Verification items for the finished model (mm, model axes). A direction names the side the tool comes from. Round coordinates to 2 decimals unless told otherwise and drop trailing zeros. Order: outer loops, then holes, each group sorted by start corner. A loop starts at its lowest first (then second) coordinate and runs counter-clockwise, first axis right, second up. Notation, with made-up numbers: M 70,63.5 L 92,63.5 A6 cw 92,74.5 Z; hole C -26,48 d4. An arc over 180 degrees is marked long. Return JSON: item names as keys, results as strings. Group by question number.
from build123d import *

# Parameters (mm, degrees)
BOSS_EXTRU_1_DEPTH      = 530
ESQUISSE2_R             = 2.5
ENL_V_MAT_EXTRU_1_DEPTH = 9


with BuildPart() as part:
    # Esquisse1 → Boss.-Extru.1 (new body)
    with BuildSketch(Plane.XY):
        Polygon((0, 0), (90, 0), (90, 7), (49.5, 7), (49.5, 60), (40.5, 60), (40.5, 7), (0, 7), align=None)
    extrude(amount=BOSS_EXTRU_1_DEPTH)

    # Esquisse2 → Enlèv. mat.-Extru.1 (cut)
    with BuildSketch(Plane.ZY.offset(-40.5)):
        with Locations(Location((80, 50, 0), (0, 0, 270))):
            Circle(ESQUISSE2_R)
        with Locations(Location((80, 26, 0), (0, 0, 90))):
            Circle(ESQUISSE2_R)
        with Locations(Location((180, 50, 0), (0, 0, 270))):
            Circle(ESQUISSE2_R)
        with Locations(Location((180, 26, 0), (0, 0, 90))):
            Circle(ESQUISSE2_R)
        with Locations(Location((280, 50, 0), (0, 0, 270))):
            Circle(ESQUISSE2_R)
        with Locations(Location((280, 26, 0), (0, 0, 90))):
            Circle(ESQUISSE2_R)
        with Locations(Location((380, 50, 0), (0, 0, 270))):
            Circle(ESQUISSE2_R)
        with Locations(Location((380, 26, 0), (0, 0, 90))):
            Circle(ESQUISSE2_R)
        with Locations(Location((480, 50, 0), (0, 0, 270))):
            Circle(ESQUISSE2_R)
        with Locations(Location((480, 26, 0), (0, 0, 90))):
            Circle(ESQUISSE2_R)
    extrude(amount=-ENL_V_MAT_EXTRU_1_DEPTH, mode=Mode.SUBTRACT)


solid = part.part
1. Cross-section at A-A (z = 33). Enter the section's corners in (x, y), plus the area to 3 significant figures.
2. Cross-section at B-B (y = 42.5). Enter the section's corners in (x, z).
3. Cross-section at C-C (x = 12). Enter the section's corners in (y, z), plus the area to 3 significant figures.
4. Go/stop test with flat-tipped pins: pin 1 (6 mm diameter, centred on y = 50, z = 280, fed in from -X); pin 2 (12 mm diameter, centred on x = 24, z = 350.5, fed in from +Y); pin 3 (4 mm diameter, centred on y = 26, z = 280, fed in from -X); pin 4 (1 mm diameter, centred on x = 67.5, z = 449, fed in from -Y). Record where each tip stops, or that it passes through.
5. Thickness scan on line 1 along Z through (x, y) = (43.5, 26); line 2 along Y through (x, z) = (44.75, 280); line 3 along X through (y, z) = (52, 202). Record the ranges inside material, lowest first. Write a range as from..to.
6. Access from +Z, -Z, +X, -X, +Y, -Y to the whole of each face (thin tool, end or side, straight path). Record for faces 1 (the face through (45, 17, 0)), 2 (the face through (70, 7, 261)), 3 (the face through (40.5, 34, 261)).
Computed:
{
 "1": {"outline": "M 0,0 L 90,0 L 90,7 L 49.5,7 L 49.5,60 L 40.5,60 L 40.5,7 L 0,7 Z", "area": "1,110 mm²"},
 "2": {"outline": "M 40.5,0 L 49.5,0 L 49.5,530 L 40.5,530 Z"},
 "3": {"outline": "M 0,0 L 7,0 L 7,530 L 0,530 Z", "area": "3,710 mm²"},
 "4": {"pin 1": "stops at x = 40.5", "pin 2": "stops at y = 7", "pin 3": "passes through", "pin 4": "stops at y = 0"},
 "5": {"line 1": "z = 0..77.5, 82.5..177.5, 182.5..277.5, 282.5..377.5, 382.5..477.5, 482.5..530", "line 2": "y = 0..23.5, 28.5..47.5, 52.5..60", "line 3": "x = 40.5..49.5"},
 "6": {"face 1": "-Z, +X, -X, +Y, -Y", "face 2": "+Z, -Z, +X, +Y", "face 3": "+Z, -Z, -X, +Y"}
}
